from build123d import *

# Parameters (mm, degrees)
SKETCH1_R             = 6.35
BOSS_EXTRUDE1_DEPTH   = 14.605
SKETCH2_R             = 1.5875
CUT_EXTRUDE1_DEPTH    = 18.145
BODY_MOVE_COPY3_ANGLE = 0.1216002


with BuildPart() as part:
    # Sketch1 → Boss-Extrude1 (new body)
    with BuildSketch(Plane(origin=(0, 0, 0), x_dir=(1, 0, 0), z_dir=(0, 1, 0))):
        with Locations(Location((0, 0, 0), (0, 0, 90))):
            Circle(SKETCH1_R)
    extrude(amount=BOSS_EXTRUDE1_DEPTH)

    # Sketch2 → Cut-Extrude1 (cut, through all)
    with BuildSketch(Plane(origin=(0, 0, 0), x_dir=(-1, 0, 0), z_dir=(0, -1, 0))):
        with Locations(Location((0, 0, 0), (0, 0, 90))):
            Circle(SKETCH2_R)
    extrude(amount=-CUT_EXTRUDE1_DEPTH, mode=Mode.SUBTRACT)

    # Sketch16 → #8-32 Tapped Hole3 (revolve, cut)
    with BuildSketch(Plane(origin=(6.349985699, 3.048, -0.013476749), x_dir=(-0.002122322633644313, 0, -0.9999977478707834), z_dir=(0, 1, 0))):
        Polygon((0, 0), (0, 9.927806461), (1.7272, 8.89), (1.7272, 0.635), (2.3622, 0), align=None)
    f_8_32_tapped_hole3 = revolve(axis=Axis((12.699971398, 3.048, -0.026953497), (-0.9999977478707834, 0, 0.002122322633644313)), mode=Mode.SUBTRACT)

    # Mirror2: #8-32 Tapped Hole3 across plane
    add(f_8_32_tapped_hole3.mirror(Plane.ZX.offset(7.3025)), mode=Mode.SUBTRACT)


with BuildPart() as part_1:
    # Body-Move/Copy3: read off the stored shape, not the designer's step
    # Body-Move/Copy3: moved
    add(part.part.moved(Location((-5.7150129, 0, 0))).rotate(Axis((0, 0, 0), (0, -1, 0)), BODY_MOVE_COPY3_ANGLE))


solid = part_1.part
The model under review builds one solid part; all positions refer to its coordinate system, in mm. A direction names the side the tool comes from. Round coordinates to 2 decimals unless told otherwise and drop trailing zeros. Order: outer loops, then holes, each group sorted by start corner. A loop starts at its lowest first (then second) coordinate and runs counter-clockwise, first axis right, second up. Notation, with made-up numbers: (88.25, 89) -> (110.25, 89) arc R14 ccw to (110.25, 108) -> close; hole circle Ø10 at (-37, 62.25). An arc over 180 degrees is marked (long way). Write item = value, one per line. Start each with the question number.
Item 1: Clearance check with a flat-ended pin moving along its axis: pin 1 Ø2 at (x, y) = (-4, 12) entering from +Z. State where the tip first meets the part, or that it passes through.
Item 2: Mouldability with a two-part tool opening along Z and no side actions: class faces 1 (the face through (-12.013, 7.2, 0.801)), 2 (the face through (-4, 0, -1)), 3 (the face through (-4.07, 3.71, -1.608)) as released by +Z, released by -Z, zero draft, split by the parting line, or undercut.
Item 3: Consider section C-C on z = 0.25. Count the separate pieces of the cut face and the enclosed holes in it, plus the area to 3 significant figures.
Item 4: Consider section B-B on x = -2.75. Write out the cut boundary in (y, z) (3 decimals), plus the area to 3 significant figures.
Item 5: For line 1 along X through (y, z) = (9, 0); line 2 along Z through (x, y) = (-10, 4); line 3 along X through (y, z) = (11, 3.25), list the stretches that pass through material, from the lowest coordinate up.
Item 6: Consider section A-A on x = -6.5. Write out the cut boundary in (y, z) (3 decimals).
Item 7: For faces 4 (the face through (-5.649, 0.904, 1.574)), 5 (the face through (-4.07, 10.9, -1.61)), list the 3-axis set-ups (+Z, -Z, +X, -X, +Y, -Y) from which the entire face can be reached by the end or side of a thin tool; tool diameter is ignored.
Conclusion:
q1.pin_1 = 6.3
q2.face_1 = split by the parting line
q2.face_2 = zero draft
q2.face_3 = undercut
q3.separate_pieces = 4
q3.enclosed_holes = 0
q3.area = 96.2 mm2
q4.outline = (0, -5.627) -> (14.605, -5.627) -> (14.605, 5.603) -> (0, 5.603) -> close; hole circle Ø3.454 at (3.048, -0.012); hole circle Ø3.454 at (11.557, -0.012)
q4.area = 145 mm2
q5.line_1 = -12.06 to -7.3, -4.13 to 0.63
q5.line_2 = -4.7 to 4.67
q5.line_3 = -11.16 to -0.27
q6.outline = (0, -6.313) -> (14.605, -6.313) -> (14.605, -1.392) -> (12.596, -1.392) arc R1.727 cw to (10.518, -1.392) -> (4.087, -1.392) arc R1.727 cw to (2.009, -1.392) -> (0, -1.392) -> close; (0, 1.368) -> (2.009, 1.368) arc R1.727 cw to (4.087, 1.368) -> (10.518, 1.368) arc R1.727 cw to (12.596, 1.368) -> (14.605, 1.368) -> (14.605, 6.289) -> (0, 6.289) -> close
q7.face_4 = +Y, -Y
q7.face_5 = +X
